Verification items for the finished model (mm, model axes). A direction names the side the tool comes from. Round coordinates to 2 decimals unless told otherwise and drop trailing zeros. Order: outer loops, then holes, each group sorted by start corner. A loop starts at its lowest first (then second) coordinate and runs counter-clockwise, first axis right, second up. Notation, with made-up numbers: (-29.75, -30) -> (9.25, -30) arc R20 cw to (9.25, -3) -> close; hole circle Ø3 at (15, 81.5). An arc over 180 degrees is marked (long way). Put each result on its own line as item: value.
```python
from build123d import *

# Parameters (mm, degrees)
SKETCH_1_W      = 55
SKETCH_1_H      = 46
EXTRUDE_1_DEPTH = 3
SKETCH_2_W      = 3
SKETCH_2_H      = 5
EXTRUDE_2_DEPTH = 2
CHAMFER_1_SIZE  = 2


with BuildPart() as part:
    # Эскиз1 → Бобышка-Вытянуть1 (new body)
    with BuildSketch(Plane.XY):
        with Locations((0, 20)):
            Rectangle(SKETCH_1_W, SKETCH_1_H)
    extrude(amount=EXTRUDE_1_DEPTH)

    # Эскиз2 → Бобышка-Вытянуть2 (add)
    with BuildSketch(Plane(origin=(0, 0, 0), x_dir=(-1, 0, 0), z_dir=(0, 0, -1))):
        with Locations((-22.6, 20)):
            Rectangle(SKETCH_2_W, SKETCH_2_H)
        with Locations((22.6, 20)):
            Rectangle(SKETCH_2_W, SKETCH_2_H)
    extrude(amount=EXTRUDE_2_DEPTH)

    # Фаска1
    chamfer_1_edges = [part.edges().sort_by_distance(p)[0] for p in [
        (-22.6, 17.5, 0),
        (-21.1, 20, 0),
        (-22.6, 22.5, 0),
        (22.6, 22.5, 0),
        (21.1, 20, 0),
        (22.6, 17.5, 0),
    ]]
    chamfer(chamfer_1_edges, length=CHAMFER_1_SIZE - 0.0001)  # a hair under: the kernel refuses the full size


solid = part.part
```
Item 1: Tool access check on faces 5 (the face through (-24.1, 20, -1)), 6 (the face through (24.1, 20, -1)), 7 (the face through (0, 43, 1)). Record the directions out of +Z, -Z, +X, -X, +Y, -Y that give a thin tool (end or side, any length) a straight path to the whole face; none if there is none.
Geometry check:
face 5: -Z, -X, +Y, -Y
face 6: -Z, +X, +Y, -Y
face 7: +Z, -Z, +X, -X, +Y
Item 2: Release check for a two-part mould opening along X. For faces 1 (the face through (20.1, 19.9, -1)), 2 (the face through (-20.1, 19.9, -1)), 3 (the face through (-27.5, 20, 1)), 4 (the face through (-23, 20, -2)) record: pulls with the +X half, pulls with the -X half, needs draft (parallel to the pull), parting line crosses it, or undercut.
Geometry check:
face 1: undercut
face 2: undercut
face 3: pulls with the -X half
face 4: needs draft
Item 3: Material ranges on line 1 along Z through (x, y) = (-16.5, 28); line 2 along Z through (x, y) = (20, 22.5); line 3 along X through (y, z) = (17.5, -1.35), recorded low to high.
Geometry check:
line 1: 0 to 3
line 2: -0.9 to 3
line 3: -24.1 to -20.45, 20.45 to 24.1
Item 4: Sectioned sample at A-A, the plane z = -1.4. Record the boundary of the cut face in (x, y).
Geometry check:
outline: (-24.1, 16.9) -> (-20.5, 16.9) -> (-20.5, 23.1) -> (-24.1, 23.1) -> close; (20.5, 16.9) -> (24.1, 16.9) -> (24.1, 23.1) -> (20.5, 23.1) -> close
Item 5: Depth check by flat-ended pin: pin 1 Ø3 at (x, y) = (6.5, 17) entering from -Z; pin 2 Ø0.6 at (y, z) = (20, -1.5) entering from -X. Enter the tip coordinate at first touch or a pass-through.
Geometry check:
pin 1: z = 0
pin 2: x = -24.1
Item 6: Sectioned sample at D-D, the plane y = 1.5. Record the boundary of the cut face in (x, z), then the cut area to 3 significant figures.
Geometry check:
outline: (-27.5, 0) -> (27.5, 0) -> (27.5, 3) -> (-27.5, 3) -> close
area: 165 mm2
